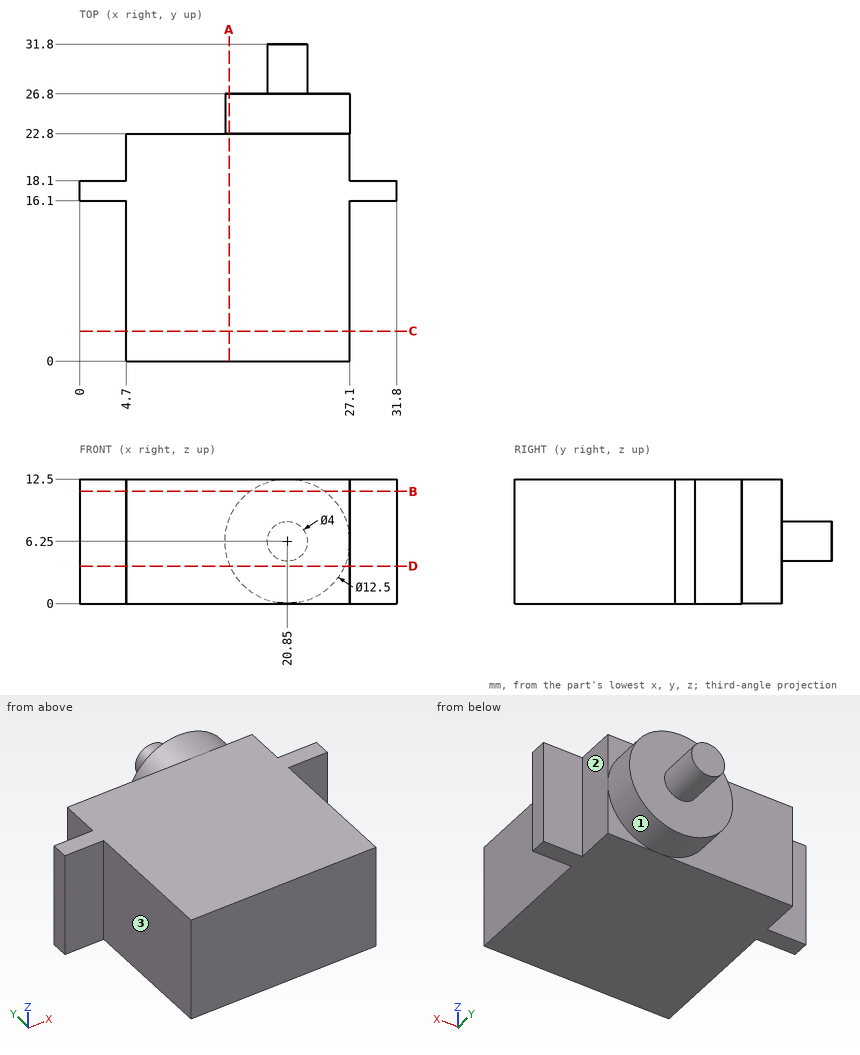
Study the drawing (mm; zero at the part's minimum x, y, z) and answer. A direction names the side the tool comes from. Round coordinates to 2 decimals unless told otherwise and drop trailing zeros. Order: outer loops, then holes, each group sorted by start corner. A loop starts at its lowest first (then second) coordinate and runs counter-clockwise, first axis right, second up. Notation, with made-up numbers: M -33.75,-39.75 L -13.75,-39.75 A11 ccw -13.75,-20.75 Z; hole C 6,-32 d10. An arc over 180 degrees is marked long. One line per item, written item: value.
Q1. Find section C-C on y = 3. Write down the section's boundary in (x, z), then the cut area to 3 significant figures.
Derived:
outline: M 4.7,0 L 27.1,0 L 27.1,12.5 L 4.7,12.5 Z
area: 280 mm²
Q2. Straight lines are drawn through the part: line 1 (X direction, y = 10.5, z = 9.25); line 2 (Y direction, x = 27, z = 5.75); line 3 (Y direction, x = 30, z = 2.5). For each, find the intervals that lie inside material, in ascending order.
Derived:
line 1: 4.7 to 27.1
line 2: 0 to 26.8
line 3: 16.1 to 18.1
Q3. Find section B-B on z = 11.25. Write down the section's boundary in (x, y).
Derived:
outline: M 0,16.1 L 4.7,16.1 L 4.7,0 L 27.1,0 L 27.1,16.1 L 31.8,16.1 L 31.8,18.1 L 27.1,18.1 L 27.1,22.8 L 24.6,22.8 L 24.6,26.8 L 17.1,26.8 L 17.1,22.8 L 4.7,22.8 L 4.7,18.1 L 0,18.1 Z
Q4. For the marked faces 1, 2 and 3, determine the directions among +Z, -Z, +X, -X, +Y, -Y from which every point of the face is accessible in a straight line to the end or side of a thin tool.
Derived:
face 1: +Y
face 2: +Z, -Z, +X, +Y
face 3: +Z, -Z, -X, -Y
Q5. Find section A-A on x = 15. Write down the section's boundary in (y, z).
Derived:
outline: M 0,0 L 22.8,0 L 22.8,4.05 L 26.8,4.05 L 26.8,8.45 L 22.8,8.45 L 22.8,12.5 L 0,12.5 Z
Q6. Find section D-D on z = 3.75. Write down the section's boundary in (x, y), then the cut area to 3 significant figures.
Derived:
outline: M 0,16.1 L 4.7,16.1 L 4.7,0 L 27.1,0 L 27.1,16.1 L 31.8,16.1 L 31.8,18.1 L 27.1,18.1 L 27.1,22.8 L 26.58,22.8 L 26.58,26.8 L 15.12,26.8 L 15.12,22.8 L 4.7,22.8 L 4.7,18.1 L 0,18.1 Z
area: 575 mm²
Q7. Flat-ended cylindrical pins translate along their axes: pin 1 (5 mm diameter, centred on x = 24, z = 10.5, fed in from +Y); pin 2 (1.4 mm diameter, centred on x = 3, z = 8.5, fed in from +Y); pin 3 (1 mm diameter, centred on y = 9.5, z = 6.5, fed in from -X). Find the tip coordinate at first contact, or state that the pin passes through.
Derived:
pin 1: y = 26.8
pin 2: y = 18.1
pin 3: x = 4.7
